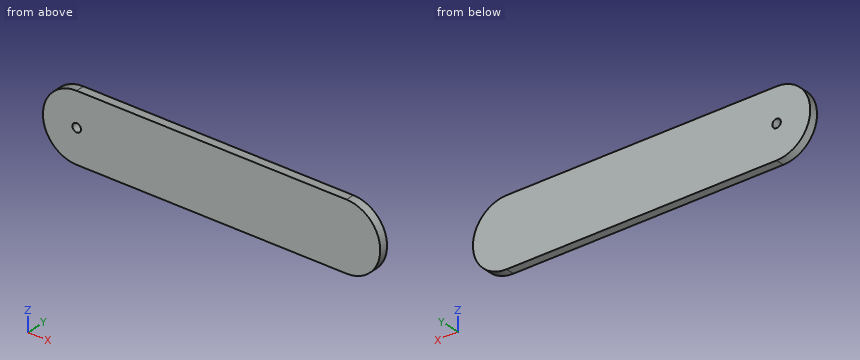
```python
from build123d import *

# Parameters (mm, degrees)
BOSS_EXTRUDE1_DEPTH = 6.35
SKETCH4_R           = 3.175
CUT_EXTRUDE1_DEPTH  = 7.35


with BuildPart() as part:
    # Sketch2 → Boss-Extrude1 (new body)
    with BuildSketch(Plane(origin=(0, 0, 0), x_dir=(1, 0, 0), z_dir=(0, 1, 0))):
        with BuildLine():
            Line((0, 25), (200, 25))
            ThreePointArc((200, 25), (225, 0), (200, -25))
            Line((200, -25), (0, -25))
            ThreePointArc((0, -25), (-25, 0), (0, 25))
        make_face()
    extrude(amount=BOSS_EXTRUDE1_DEPTH)

    # Sketch4 → Cut-Extrude1 (cut, through all)
    with BuildSketch(Plane(origin=(0, 6.35, 0), x_dir=(1, 0, 0), z_dir=(0, 1, 0))):
        Circle(SKETCH4_R)
    extrude(amount=-CUT_EXTRUDE1_DEPTH, mode=Mode.SUBTRACT)


solid = part.part
```
Geometry: final body of the model. Coordinates: model frame, mm. Round coordinates to 2 decimals unless told otherwise and drop trailing zeros. Order: outer loops, then holes, each group sorted by start corner. A loop starts at its lowest first (then second) coordinate and runs counter-clockwise, first axis right, second up. Notation, with made-up numbers: M -24,11.5 L 7,11.5 A24 ccw 7,43.5 Z; hole C 37,10 d7. An arc over 180 degrees is marked long. Use one line per item in the form item = value. Start each with the question number.
Q1. Pin query (flat end, axial travel): pin 1 Ø2 at (y, z) = (3.5, 1) entering from -X; pin 2 Ø4 at (x, z) = (0, 0) entering from -Y; pin 3 Ø6 at (x, z) = (130.5, -18) entering from -Y. Return the tip coordinate at first contact, or that it passes through.
Q2. Cut plane D-D (z = -10). Return loops of the section in (x, y).
Q3. Cut plane A-A (z = 0). Return loops of the section in (x, y) (3 decimals).
Q4. Cut plane B-B (y = 1.5). Return loops of the section in (x, z) (3 decimals).
Q5. Material intervals for line 1 (X direction, y = 3.5, z = 0) (3 decimals); line 2 (Z direction, x = 0, y = 4.75) (3 decimals); line 3 (X direction, y = 2.5, z = -1), sorted ascending. Write a range as [from, to].
Q6. Cut plane C-C (z = 11.5). Return loops of the section in (x, y).
Geometry results:
q1.pin_1 = -25
q1.pin_2 = through
q1.pin_3 = 0
q2.outline = M -22.91,0 L 222.91,0 L 222.91,6.35 L -22.91,6.35 Z
q3.outline = M -25,0 L -3.175,0 L -3.175,6.35 L -25,6.35 Z; M 3.175,0 L 225,0 L 225,6.35 L 3.175,6.35 Z
q4.outline = M 0,-25 L 200,-25 A25 ccw 200,25 L 0,25 A25 ccw Z; hole C 0,0 d6.35
q5.line_1 = [-25, -3.175], [3.175, 225]
q5.line_2 = [-25, -3.175], [3.175, 25]
q5.line_3 = [-24.98, -3.01], [3.01, 224.98]
q6.outline = M -22.2,0 L 222.2,0 L 222.2,6.35 L -22.2,6.35 Z
